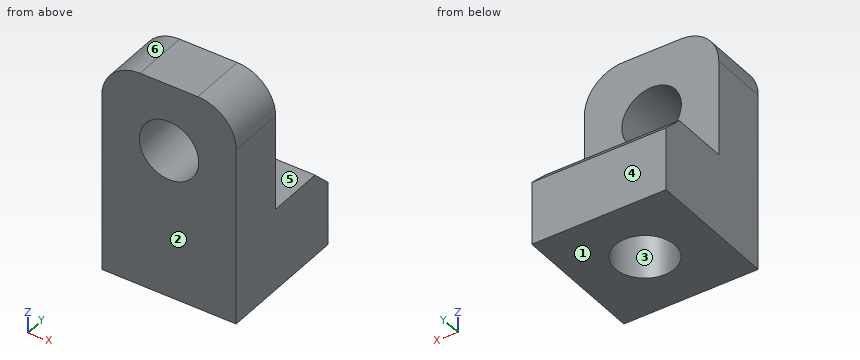
```python
from build123d import *

# Parameters (mm, degrees)
SKETCH1_W           = 7
SKETCH1_H           = 7
SKETCH1_R           = 1.55
BOSS_EXTRUDE1_DEPTH = 2.3
SKETCH3_W           = 7
SKETCH3_H           = 7
BOSS_EXTRUDE2_DEPTH = 2
SKETCH4_W           = 7
SKETCH4_H           = 3
BOSS_EXTRUDE3_DEPTH = 7
CUT_EXTRUDE1_REACH  = 9
SKETCH5_R           = 1.55
FILLET1_R           = 2
CHAMFER1_SIZE       = 1


with BuildPart() as part:
    # Sketch1 → Boss-Extrude1 (new body)
    with BuildSketch(Plane.XY):
        with Locations((5, 6.5)):
            Rectangle(SKETCH1_W, SKETCH1_H)
        with Locations((5, 6.5)):
            Circle(SKETCH1_R, mode=Mode.SUBTRACT)
    extrude(amount=BOSS_EXTRUDE1_DEPTH)

    # Sketch3 → Boss-Extrude2 (add)
    with BuildSketch(Plane.XY.offset(2.3)):
        with Locations((5, 6.5)):
            Rectangle(SKETCH3_W, SKETCH3_H)
    extrude(amount=BOSS_EXTRUDE2_DEPTH)

    # Sketch4 → Boss-Extrude3 (add)
    with BuildSketch(Plane.XY.offset(4.3)):
        with Locations((5, 4.5)):
            Rectangle(SKETCH4_W, SKETCH4_H)
    extrude(amount=BOSS_EXTRUDE3_DEPTH)

    # Sketch5 → Cut-Extrude1 (cut, up to next)
    with BuildSketch(Plane.XZ.offset(-3), mode=Mode.PRIVATE) as cut_extrude1_sk1:
        with Locations((5, 7.8)):
            Circle(SKETCH5_R)
    cut_extrude1_tool1 = extrude(cut_extrude1_sk1.sketch, amount=-CUT_EXTRUDE1_REACH, mode=Mode.PRIVATE) & part.part
    add(cut_extrude1_tool1.solids().sort_by_distance((5, 3, 7.8))[0], mode=Mode.SUBTRACT)

    # Fillet1
    fillet1_edges = [part.edges().sort_by_distance(p)[0] for p in [
        (8.5, 4.5, 11.3),
        (1.5, 4.5, 11.3),
    ]]
    fillet(fillet1_edges, radius=FILLET1_R)

    # Chamfer1
    chamfer1_edges = [part.edges().sort_by_distance(p)[0] for p in [
        (5, 10, 4.3),
    ]]
    chamfer(chamfer1_edges, length=CHAMFER1_SIZE)


solid = part.part
```
Geometry: final body of the model. Coordinates: model frame, mm. Face numbers are marked on the shaded views. A direction names the side the tool comes from. Give positions to 0.01 mm unless a question says otherwise; leave off trailing zeros. Write each loop counter-clockwise with the first axis right and the second up, starting at its lowest first coordinate (ties: lowest second). Pieces come first, ordered by that corner, then holes.
1. Draft query along Y for the marked faces 1, 2, 3 and 4. Return one class per face: released by +Y, released by -Y, zero draft, split by the parting line, or undercut.
2. Reachability of the marked faces 5 and 6 from +Z, -Z, +X, -X, +Y, -Y: full face, straight path, thin tool, end or side. Return the list, or none.
3. Line query: probe 1 along Z at (x, y) = (5, 3.6); probe 2 along Y at (x, z) = (5, 0.95); probe 3 along Z at (x, y) = (6.25, 7.25). Output: solid intervals per line, ascending.
4. Section query A-A, the plane z = 7.8. Return loops of the section in (x, y), then the cut area to 3 significant figures.
5. Section query C-C, the plane x = 5. Return loops of the section in (y, z).
6. Section query B-B, the plane y = 4.25. Return loops of the section in (x, z).
7. Section query D-D, the plane y = 6.5. Return loops of the section in (x, z).
Computed:
1. face 1: zero draft
1. face 2: released by -Y
1. face 3: undercut
1. face 4: released by +Y
2. face 5: +Z, +X, -X, +Y
2. face 6: +Z, -X, +Y, -Y
3. probe 1: z = 0 to 6.25, 9.35 to 11.3
3. probe 2: y = 3 to 4.95, 8.05 to 10
3. probe 3: z = 2.3 to 4.3
4. outline: (1.5, 3) - (3.45, 3) - (3.45, 6) - (1.5, 6) - close; (6.55, 3) - (8.5, 3) - (8.5, 6) - (6.55, 6) - close
4. area: 11.7 mm2
5. outline: (3, 0) - (4.95, 0) - (4.95, 2.3) - (8.05, 2.3) - (8.05, 0) - (10, 0) - (10, 3.3) - (9, 4.3) - (6, 4.3) - (6, 6.25) - (3, 6.25) - close; (3, 9.35) - (6, 9.35) - (6, 11.3) - (3, 11.3) - close
6. outline: (1.5, 0) - (8.5, 0) - (8.5, 9.3) arc R2 ccw to (6.5, 11.3) - (3.5, 11.3) arc R2 ccw to (1.5, 9.3) - close; hole circle Ø3.1 at (5, 7.8)
7. outline: (1.5, 0) - (3.45, 0) - (3.45, 2.3) - (6.55, 2.3) - (6.55, 0) - (8.5, 0) - (8.5, 4.3) - (1.5, 4.3) - close
